```python
from build123d import *

# Parameters (mm, degrees)
F2_DEPTH = 25
F4_D     = 9
F6_D     = 9


with BuildPart() as f2:
    # F1 (on offset) → F2 (new body)
    with BuildSketch(Plane.YZ.offset(60)):
        with BuildLine():
            ThreePointArc((-12.5, 0), (0, 12.5), (12.5, 0))
            Line((12.5, 0), (12.5, -120))
            Line((12.5, -120), (17.5, -120))
            Line((17.5, -120), (17.5, 0))
            ThreePointArc((17.5, 0), (0, 17.5), (-17.5, 0))
            Line((-17.5, 0), (-12.5, 0))
        make_face()
    extrude(amount=-F2_DEPTH)

    # F4 (through all)
    with Locations(Plane(origin=(0, 17.5, 0), x_dir=(-1, 0, 0), z_dir=(0, 1, 0))):
        with Locations((-47.5, -25), (-47.5, -45)):
            Hole(F4_D / 2)

    # F6 (through all)
    with Locations(Plane(origin=(0, 17.5, 0), x_dir=(-1, 0, 0), z_dir=(0, 1, 0))):
        with Locations((-47.5, -75), (-47.5, -95)):
            Hole(F6_D / 2)


solid = f2.part
```
Geometry: final body of the model. Coordinates: model frame, mm. A direction names the side the tool comes from. Coordinates: 2 decimals unless noted, no trailing zeros. Write each loop counter-clockwise with the first axis right and the second up, starting at its lowest first coordinate (ties: lowest second). Pieces come first, ordered by that corner, then holes. Notation, with made-up numbers: M 18.25,-22.5 L 54.25,-22.5 A24 ccw 54.25,15.5 Z; hole C 68,-20.5 d5. An arc over 180 degrees is marked long. Answer as CSV lines item,"result". Start each with the question number.
Q1. Line query: line 1 (Z direction, x = 47.5, y = 14.35); line 2 (Z direction, x = 47.5, y = 15.15); line 3 (Y direction, x = 39.5, z = -71). Output: solid intervals per line, ascending. Write a range as from..to.
Q2. Reachability of faces 1 (the flat face through (48, -15, 0)), 2 (the flat face through (60, 13, -41)) from +Z, -Z, +X, -X, +Y, -Y: full face, straight path, thin tool, end or side. Return the list, or none.
Q3. Cut plane D-D on y = 0. Return the cut outline in (x, z).
Q4. Cut plane A-A on x = 47.5. Return the cut outline in (y, z).
Q5. Mould query, pull axis Y, two halves, no side actions, for faces 3 (the flat face through (48, 17.5, -61)), 4 (the cylindrical face through (47.675, -0.275, 12.497)), 5 (the cylindrical face through (49.58, 14.97, -48.99)). Classes: released by +Y, released by -Y, zero draft, split by the parting line, or undercut.
Q6. Cut plane B-B on z = -45. Return the cut outline in (x, y).
Q7. Pin query (flat end, axial travel): P1, Ø8, axis at x = 50, z = -26.5, coming from the -Y side; P2, Ø2, axis at x = 49.5, y = 9.5, coming from the -Z side; P3, Ø7, axis at x = 47.5, z = -25, coming from the -Y side; P4, Ø4, axis at x = 48.5, y = 3.5, coming from the +Z side. Return the tip coordinate at first contact, or that it passes through.
Q8. Cut plane C-C on x = 53.5. Return the cut outline in (y, z).
Findings below:
1,line 1,"z = -120..-99.5, -90.5..-79.5, -70.5..-49.5, -40.5..-29.5, -20.5..10.02"
1,line 2,"z = -120..-99.5, -90.5..-79.5, -70.5..-49.5, -40.5..-29.5, -20.5..8.76"
1,line 3,"y = 12.5..17.5"
2,face 1,"-Z, +X, -X, -Y"
2,face 2,"+Z, -Z, +X, +Y, -Y"
3,outline,"M 35,12.5 L 60,12.5 L 60,17.5 L 35,17.5 Z"
4,outline,"M -17.5,0 L -12.5,0 A12.5 cw 12.5,0 L 12.5,-20.5 L 17.5,-20.5 L 17.5,0 A17.5 ccw Z; M 12.5,-120 L 17.5,-120 L 17.5,-99.5 L 12.5,-99.5 Z; M 12.5,-90.5 L 17.5,-90.5 L 17.5,-79.5 L 12.5,-79.5 Z; M 12.5,-70.5 L 17.5,-70.5 L 17.5,-49.5 L 12.5,-49.5 Z; M 12.5,-40.5 L 17.5,-40.5 L 17.5,-29.5 L 12.5,-29.5 Z"
5,face 3,"released by +Y"
5,face 4,"undercut"
5,face 5,"zero draft"
6,outline,"M 35,12.5 L 43,12.5 L 43,17.5 L 35,17.5 Z; M 52,12.5 L 60,12.5 L 60,17.5 L 52,17.5 Z"
7,P1,"stops at y = 12.5"
7,P2,"stops at z = 6.78"
7,P3,"passes through"
7,P4,"stops at z = 17.44"
8,outline,"M -17.5,0 L -12.5,0 A12.5 cw 12.5,0 L 12.5,-120 L 17.5,-120 L 17.5,0 A17.5 ccw Z"
